Study the drawing (mm; zero at the part's minimum x, y, z) and answer. A direction names the side the tool comes from. Coordinates: 2 decimals unless noted, no trailing zeros. Loops run counter-clockwise (first coordinate to the right, second up) from the corner with the lowest first, then second, coordinate; pieces in that order, holes last. Notation, with made-up numbers: (61.25, -34.75) - (82.25, -34.75) arc R26 cw to (82.25, -16.75) - close; hole circle Ø5 at (49, 25). An arc over 180 degrees is marked (long way). Use CSV: the item, a comma, the result in double quotes.
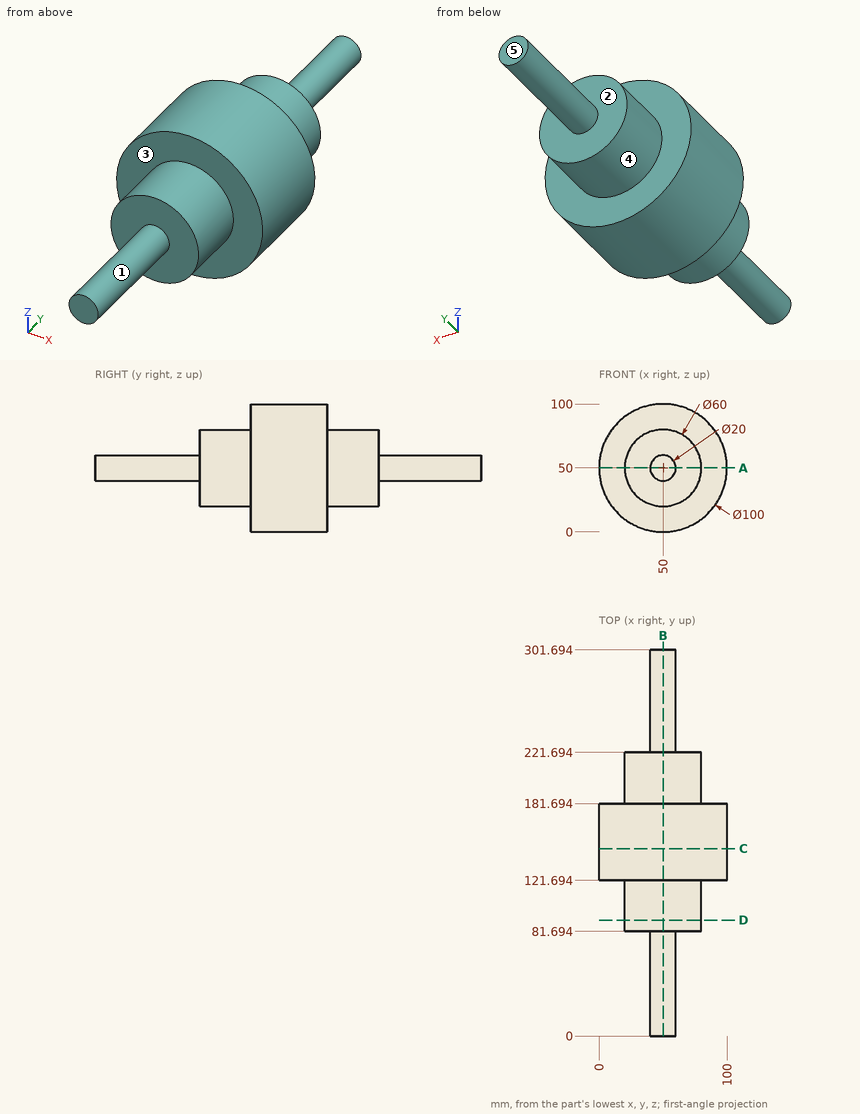
Q1. The part is cut by section B-B on x = 50. Determine the outline of the cut face in (y, z), and give its area (3 significant figures).
Reported:
outline,"(0, 40) - (81.69, 40) - (81.69, 20) - (121.69, 20) - (121.69, 0) - (181.69, 0) - (181.69, 20) - (221.69, 20) - (221.69, 40) - (301.69, 40) - (301.69, 60) - (221.69, 60) - (221.69, 80) - (181.69, 80) - (181.69, 100) - (121.69, 100) - (121.69, 80) - (81.69, 80) - (81.69, 60) - (0, 60) - close"
area,"14,000 mm²"
Q2. The part is cut by section D-D on y = 90.5. Determine the outline of the cut face in (x, z), and give its area (3 significant figures).
Reported:
outline,"circle Ø60 at (50, 50)"
area,"2,830 mm²"
Q3. For a pull along X with two mould halves and no side action, classify the marked faces 1 and 2 as +X half, -X half, draft (parallel to the pull), parting line (faces both ways), or undercut.
Reported:
face 1,"parting line"
face 2,"draft"
Q4. A tool of negligible diameter and unlimited length cuts with its end or side. For the marked faces 3, 4 and 5, from which of +Z, -Z, +X, -X, +Y, -Y can it reach the whole face along a straight path? Write none if from no direction.
Reported:
face 3,"-Y"
face 4,"+Y"
face 5,"+Z, -Z, +X, -X, +Y"
Q5. Find the intervals of material crossed by probe 1 along Y at (x, z) = (36, 6); probe 2 along Z at (x, y) = (50.5, 17.5); probe 3 along X at (y, z) = (195, 54.5), in increasing order. Write a range as [from, to].
Reported:
probe 1,"y = [121.69, 181.69]"
probe 2,"z = [40.01, 59.99]"
probe 3,"x = [20.34, 79.66]"
Q6. The part is cut by section A-A on z = 50. Determine the outline of the cut face in (x, y), and give its area (3 significant figures).
Reported:
outline,"(0, 121.69) - (20, 121.69) - (20, 81.69) - (40, 81.69) - (40, 0) - (60, 0) - (60, 81.69) - (80, 81.69) - (80, 121.69) - (100, 121.69) - (100, 181.69) - (80, 181.69) - (80, 221.69) - (60, 221.69) - (60, 301.69) - (40, 301.69) - (40, 221.69) - (20, 221.69) - (20, 181.69) - (0, 181.69) - close"
area,"14,000 mm²"
Q7. The part is cut by section C-C on y = 146.5. Determine the outline of the cut face in (x, z).
Reported:
outline,"circle Ø100 at (50, 50)"
Q8. Given P1, Ø4, axis at y = 162, z = 22.5, coming from the -X side; P2, Ø4, axis at x = 27, y = 88.5, coming from the -Z side; P3, Ø3, axis at y = 96, z = 55, coming from the +X side, each flat-ended and moving along its own axis, determine where each tip first touches the part or whether it passes through.
Reported:
P1,"stops at x = 6.99"
P2,"stops at z = 28.58"
P3,"stops at x = 79.8"
